Could you check a few things on this model? Use its own coordinates, in mm. Coordinates: 2 decimals unless noted, no trailing zeros. Order: outer loops, then holes, each group sorted by start corner. A loop starts at its lowest first (then second) coordinate and runs counter-clockwise, first axis right, second up. Notation, with made-up numbers: (76.25, -38) - (86.25, -38) arc R25 cw to (86.25, -8) - close; hole circle Ø7 at (-8, -10). An arc over 180 degrees is marked (long way). Answer as a JSON object with one key per item and string values. Group by question number.
(1) Please list where these lines run through material, in increasing order: probe 1 along Y at (x, z) = (-95.25, 12); probe 2 along Y at (x, z) = (0, 10); probe 3 along X at (y, z) = (63.5, 12).
(2) Will this pin go through, and if not, where does the flat tip stop? P1, Ø5, axis at x = 1, y = -1.5, coming from the -Z side.
(3) Imagine slicing it at B-B, the plane x = 76.2. Write out the boundary of the cut face in (y, z), and give its area (3 significant figures).
(4) Imagine slicing it at A-A, the plane x = -95.25. Write out the boundary of the cut face in (y, z).
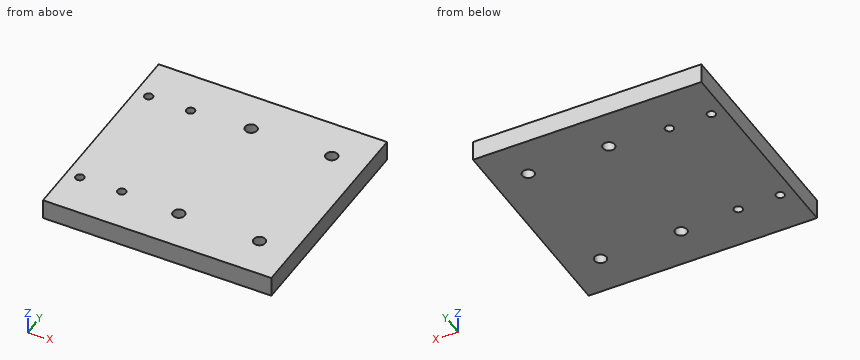
from build123d import *

# Parameters (mm, degrees)
F0_W     = 215.9
F0_H     = 203.2
F1_DEPTH = 19.05
F2_D     = 11.176
F4_D     = 7.9375


with BuildPart() as f1:
    # F0 (on Top) → F1 (new body)
    with BuildSketch(Plane.XY):
        Rectangle(F0_W, F0_H)
    extrude(amount=F1_DEPTH)

    # F2 (through all)
    with Locations(Plane(origin=(0, 0, 0), x_dir=(1, 0, 0), z_dir=(0, 0, -1))):
        with Locations((0, -63.5), (76.2, -63.5), (0, 63.5), (76.2, 63.5)):
            Hole(F2_D / 2)

    # F4 (through all)
    with Locations(Plane.XY.offset(19.05)):
        with Locations((-95.25, 60.452), (-55.626, 60.452), (-95.25, -60.452), (-55.626, -60.452)):
            Hole(F4_D / 2)


solid = f1.part
Result set:
{
 "1": {"probe 1": "y = -101.6 to -64.42, -56.48 to 56.48, 64.42 to 101.6", "probe 2": "y = -101.6 to -69.09, -57.91 to 57.91, 69.09 to 101.6", "probe 3": "x = -107.95 to -97.79, -92.71 to -58.17, -53.08 to -5.59, 5.59 to 70.61, 81.79 to 107.95"},
 "2": {"P1": "stops at z = 0"},
 "3": {"outline": "(-101.6, 0) - (-69.09, 0) - (-69.09, 19.05) - (-101.6, 19.05) - close; (-57.91, 0) - (57.91, 0) - (57.91, 19.05) - (-57.91, 19.05) - close; (69.09, 0) - (101.6, 0) - (101.6, 19.05) - (69.09, 19.05) - close", "area": "3,450 mm^2"},
 "4": {"outline": "(-101.6, 0) - (-64.42, 0) - (-64.42, 19.05) - (-101.6, 19.05) - close; (-56.48, 0) - (56.48, 0) - (56.48, 19.05) - (-56.48, 19.05) - close; (64.42, 0) - (101.6, 0) - (101.6, 19.05) - (64.42, 19.05) - close"}
}
